```python
from build123d import *

# Parameters (mm, degrees)
SKETCH_1_R             = 3.25
SM_BASE_FLANGE_1_DEPTH = 4


# Sheet-metal steps are written as plain solids
with BuildPart() as part:
    # Sketch 1 → Базовая кромка1 (new body)
    with BuildSketch(Plane.XY):
        with BuildLine():
            Line((-82.501667048, 0), (-47.907304338, -21.407039383))
            ThreePointArc((-47.907304338, -21.407039383), (-41.250833524, -23.3), (-34.594362709, -21.407039383))
            Line((-34.594362709, -21.407039383), (0, 0))
            Line((0, 0), (-82.501667048, 0))
        make_face()
        with Locations((-41.250833524, -10.65)):
            Circle(SKETCH_1_R, mode=Mode.SUBTRACT)
    extrude(amount=-SM_BASE_FLANGE_1_DEPTH)


solid = part.part
```
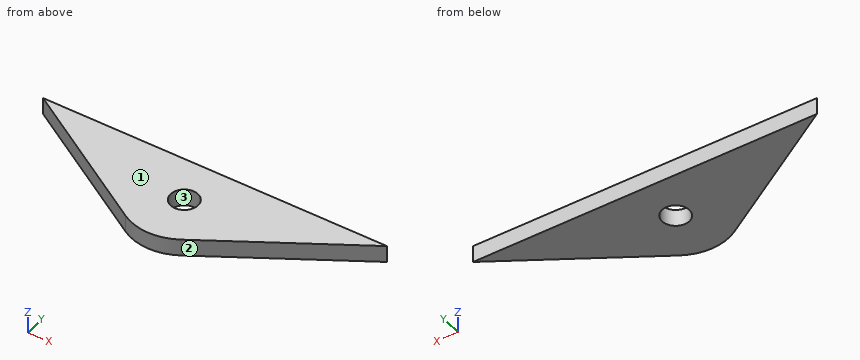
Can you work these out from the model? Positions are in its coordinate system, mm. Face numbers are marked on the shaded views. Coordinates: 2 decimals unless noted, no trailing zeros. Order: outer loops, then holes, each group sorted by start corner. A loop starts at its lowest first (then second) coordinate and runs counter-clockwise, first axis right, second up. Notation, with made-up numbers: (-27.5, 49.25) - (19.5, 49.25) arc R13 ccw to (19.5, 73.25) - close; hole circle Ø1 at (60.5, 71.5). An arc over 180 degrees is marked (long way). Answer in a Markdown table with one row per item.
1. Suppose I cut it at B-B (z = -1.1). Please give me the cut outline in (x, y), and give its area (3 significant figures).
Reply:
| item | result |
|---|---|
| outline | (-82.5, 0) - (-47.91, -21.41) arc R12.65 ccw to (-34.59, -21.41) - (0, 0) - close; hole circle Ø6.5 at (-41.25, -10.65) |
| area | 1,010 mm^2 |
2. Suppose I cut it at C-C (x = -55.5). Please give me the cut outline in (y, z).
Reply:
| item | result |
|---|---|
| outline | (-16.71, -4) - (0, -4) - (0, 0) - (-16.71, 0) - close |
3. If we mould it in two halves opening along Y, with no side actions, what happens to the marked faces 1, 2 and 3? For each: pulls with the +Y half, pulls with the -Y half, needs draft (parallel to the pull), parting line crosses it, or undercut.
Reply:
| item | result |
|---|---|
| face 1 | needs draft |
| face 2 | pulls with the -Y half |
| face 3 | undercut |
4. Suppose I cut it at A-A (y = -10.65). Please give me the cut outline in (x, z), and give its area (3 significant figures).
Reply:
| item | result |
|---|---|
| outline | (-65.29, -4) - (-44.5, -4) - (-44.5, 0) - (-65.29, 0) - close; (-38, -4) - (-17.21, -4) - (-17.21, 0) - (-38, 0) - close |
| area | 166 mm^2 |
5. If I drill on line 1 along Y through (x, z) = (-41, -0.5); line 2 along X through (y, z) = (-16.5, -0.3); line 3 along Y through (x, z) = (-31, -2.25), over which ranges is the centre line in solid material (lowest first)?
Reply:
| item | result |
|---|---|
| line 1 | y = -23.3 to -13.89, -7.41 to 0 |
| line 2 | x = -55.84 to -26.66 |
| line 3 | y = -19.18 to 0 |
6. Suppose I cut it at D-D (y = -5). Please give me the cut outline in (x, z), and give its area (3 significant figures).
Reply:
| item | result |
|---|---|
| outline | (-74.42, -4) - (-8.08, -4) - (-8.08, 0) - (-74.42, 0) - close |
| area | 265 mm^2 |
